The drawing under review shows one solid part. Ordinate dimensions are in mm from its lowest x, y, z. A direction names the side the tool comes from. Round coordinates to 2 decimals unless told otherwise and drop trailing zeros. Order: outer loops, then holes, each group sorted by start corner. A loop starts at its lowest first (then second) coordinate and runs counter-clockwise, first axis right, second up. Notation, with made-up numbers: M 76,79.25 L 121,79.25 A20 ccw 121,84.25 Z; hole C 27,10.5 d9. An arc over 180 degrees is marked long. Use a Markdown table: item, result.
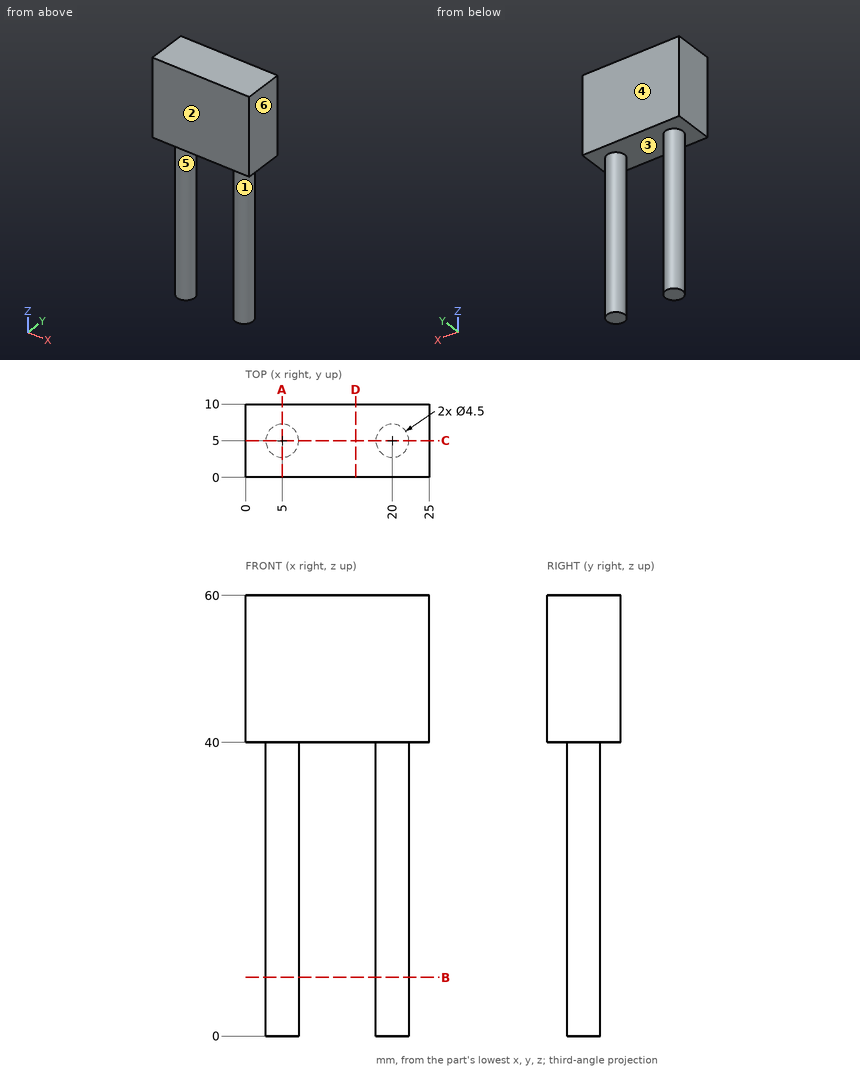
Q1. Draft analysis for pull direction X (two halves, no side actions). For the marked faces 3, 4, 5 and 6, state which applies: pulls with the +X half, pulls with the -X half, needs draft (parallel to the pull), parting line crosses it, or undercut.
Determined:
| item | result |
|---|---|
| face 3 | undercut |
| face 4 | needs draft |
| face 5 | undercut |
| face 6 | pulls with the +X half |
Q2. Wall thickness on line 1 along X through (y, z) = (3.5, 32); line 2 along X through (y, z) = (5.5, 4); line 3 along Z through (x, y) = (13, 3.5): over which ranges is each line inside the solid? List them lowest first. Write a range as [from, to].
Determined:
| item | result |
|---|---|
| line 1 | x = [3.32, 6.68], [18.32, 21.68] |
| line 2 | x = [2.81, 7.19], [17.81, 22.19] |
| line 3 | z = [40, 60] |
Q3. Add section C-C (y = 5). Write out the cut boundary in (x, z), then the cut area to 3 significant figures.
Determined:
| item | result |
|---|---|
| outline | M 0,40 L 2.75,40 L 2.75,0 L 7.25,0 L 7.25,40 L 17.75,40 L 17.75,0 L 22.25,0 L 22.25,40 L 25,40 L 25,60 L 0,60 Z |
| area | 860 mm^2 |
Q4. Add section B-B (z = 8). Write out the cut boundary in (x, y), then the cut area to 3 significant figures.
Determined:
| item | result |
|---|---|
| outline | C 5,5 d4.5; C 20,5 d4.5 |
| area | 31.8 mm^2 |
Q5. Machinability: for the marked faces 1 and 2, which of the approach directions +Z, -Z, +X, -X, +Y, -Y give a long, thin tool a straight path to every point of the face, cutting with its end or side? Answer none if there is none.
Determined:
| item | result |
|---|---|
| face 1 | -Z |
| face 2 | +Z, -Z, +X, -X, -Y |
Q6. Clearance check with flat-ended pins moving along their axes: pin 1 (3 mm diameter, centred on x = 10, y = 2.5, fed in from -Z); pin 2 (5 mm diameter, centred on x = 14.5, z = 22, fed in from -Y); pin 3 (2 mm diameter, centred on x = 22, z = 19, fed in from -Y); pin 4 (1.5 mm diameter, centred on y = 3.5, z = 36.5, fed in from -X). State where each tip first meets the part, or that it passes through.
Determined:
| item | result |
|---|---|
| pin 1 | stops at z = 40 |
| pin 2 | passes through |
| pin 3 | stops at y = 2.98 |
| pin 4 | stops at x = 2.88 |
Q7. Add section A-A (x = 5). Write out the cut boundary in (y, z).
Determined:
| item | result |
|---|---|
| outline | M 0,40 L 2.75,40 L 2.75,0 L 7.25,0 L 7.25,40 L 10,40 L 10,60 L 0,60 Z |
Q8. Add section D-D (x = 15). Write out the cut boundary in (y, z).
Determined:
| item | result |
|---|---|
| outline | M 0,40 L 10,40 L 10,60 L 0,60 Z |
